from build123d import *

# Parameters (mm, degrees)
BOSS_EXTRUDE1_DEPTH = 8.6
FILLET1_R           = 10


with BuildPart() as part:
    # Sketch1 → Boss-Extrude1 (new body)
    with BuildSketch(Plane(origin=(0, 0, 0), x_dir=(0, 0, -1), z_dir=(1, 0, 0))):
        Polygon((-20.418398158, -27.648727352), (93.581601842, -27.648727352), (93.592230689, 145.071272648), (20.221601872, 145.071272648), align=None)
        Polygon((93.581601842, -27.648727352), (93.592230689, -75.908727352), (12.587404818, -75.908727352), (-20.418398158, -27.648727352), align=None)
    extrude(amount=BOSS_EXTRUDE1_DEPTH)

    # Fillet1
    # the kernel refuses this fillet: 10 mm, written as the material it takes off along each edge
    with BuildSketch(Plane(origin=(8.6, -96.341008807, -26.561376141), x_dir=(0, 0.5645185114814042, -0.825420408152609), z_dir=(0, 0.825420408152609, 0.5645185114814043))) as fillet1_piece_1:
        with BuildLine():
            CenterArc((9.901515036, 10), FILLET1_R, 188.047846247, 81.952153753)
            Line((0, 8.6), (-0.198030301, 8.572))
            ThreePointArc((-0.198030301, 8.572), (-0.2, 4.3), (-0.2, 0))
            Line((-0.2, 0), (0, -0.2))
            Line((0, -0.2), (9.901515036, -0.2))
            Line((9.901515036, -0.2), (9.901515036, 0))
        make_face()
    extrude(amount=107.974750842, mode=Mode.SUBTRACT)
    with BuildSketch(Plane(origin=(8.6, 169.167034468, -25.891192892), x_dir=(0, -0.22903933388604258, -0.9734171682958124), z_dir=(0, -0.9734171682958125, 0.22903933388604258))) as fillet1_piece_2:
        with BuildLine():
            CenterArc((9.901515036, -10), FILLET1_R, 90, 81.952153753)
            Line((0, -8.6), (-0.198030301, -8.572))
            ThreePointArc((-0.198030301, -8.572), (-0.2, -4.3), (-0.2, 0))
            Line((-0.2, 0), (0, 0.2))
            Line((0, 0.2), (9.901515036, 0.2))
            Line((9.901515036, 0.2), (9.901515036, 0))
        make_face()
    extrude(amount=226.944347022, mode=Mode.SUBTRACT)


solid = part.part
Can you work these out from the model? Positions are in its coordinate system, mm. Round coordinates to 2 decimals unless told otherwise and drop trailing zeros. Write each loop counter-clockwise with the first axis right and the second up, starting at its lowest first coordinate (ties: lowest second). Pieces come first, ordered by that corner, then holes. Notation, with made-up numbers: M -36,35 L 13,35 A30 ccw 13,60 Z; hole C 84,-23.5 d11. An arc over 180 degrees is marked long. Use a Markdown table: item, result.
Item 1: I want a section at A-A (x = 3.25). List the corners of the cut face in (y, z) for me, and give its area (3 significant figures).
Found:
| item | result |
|---|---|
| outline | M -75.91,-93.59 L -27.65,-93.58 L 145.07,-93.59 L 145.07,-21.3 L -27.44,19.29 L -75.91,-13.86 Z |
| area | 20,600 mm2 |
Item 2: If I drill on line 1 along Z through (x, y) = (7.5, 81); line 2 along Z through (x, y) = (4.5, 0); line 3 along X through (y, z) = (-21, 13), over which ranges is the centre line in solid material (lowest first)? Write a range as [from, to].
Found:
| item | result |
|---|---|
| line 1 | z = [-93.59, -10.63] |
| line 2 | z = [-93.58, 12.04] |
| line 3 | x = [0, 7.67] |
Item 3: For pin 1 Ø4 at (x, y) = (1.5, -52.5) entering from +Z; pin 2 Ø12 at (y, z) = (62, 3) entering from -X; pin 3 Ø4 at (x, y) = (6, -43.5) entering from +Z, each with a flat end and sliding along its axis, tell me the tip position at first contact or that it passes through.
Found:
| item | result |
|---|---|
| pin 1 | stops at z = 4.53 |
| pin 2 | stops at x = 0 |
| pin 3 | stops at z = 8.27 |
